```python
from build123d import *

# Parameters (mm, degrees)
SKETCH1_R           = 1.5
SKETCH1_W           = 3
SKETCH1_H           = 3
SKETCH1_W_2         = 94
SKETCH1_H_2         = 20
SKETCH1_H_3         = 10
BOSS_EXTRUDE1_DEPTH = 3


with BuildPart() as part:
    # Sketch1 → Boss-Extrude1 (new body)
    with BuildSketch(Plane(origin=(0, 0, 0), x_dir=(1, 0, 0), z_dir=(0, 1, 0))):
        with BuildLine():
            Line((256, 103), (256, 153))
            Line((256, 153), (253, 153))
            Line((253, 153), (253, 203))
            Line((253, 203), (256, 203))
            Line((256, 203), (256, 237))
            Line((256, 237), (263, 237))
            ThreePointArc((263, 237), (265.121320344, 237.878679656), (266, 240))
            Line((266, 240), (266, 244))
            ThreePointArc((266, 244), (265.121320344, 246.121320344), (263, 247))
            Line((263, 247), (253, 247))
            Line((253, 247), (203, 247))
            Line((203, 247), (203, 250))
            Line((203, 250), (153, 250))
            Line((153, 250), (153, 247))
            Line((153, 247), (103, 247))
            Line((103, 247), (103, 250))
            Line((103, 250), (53, 250))
            Line((53, 250), (53, 247))
            Line((53, 247), (0, 247))
            Line((0, 247), (0, 200))
            Line((0, 200), (3, 200))
            Line((3, 200), (3, 150))
            Line((3, 150), (0, 150))
            Line((0, 150), (0, 100))
            Line((0, 100), (3, 100))
            Line((3, 100), (3, 50))
            Line((3, 50), (0, 50))
            Line((0, 50), (0, 0))
            Line((0, 0), (53, 0))
            Line((53, 0), (53, -3))
            Line((53, -3), (103, -3))
            Line((103, -3), (103, 0))
            Line((103, 0), (153, 0))
            Line((153, 0), (153, -3))
            Line((153, -3), (203, -3))
            Line((203, -3), (203, 0))
            Line((203, 0), (253, 0))
            Line((253, 0), (253, -3))
            Line((253, -3), (256, -3))
            Line((256, -3), (256, 0))
            Line((256, 0), (256, 43))
            Line((256, 43), (262.1, 43))
            Line((262.1, 43), (262.1, 21))
            ThreePointArc((262.1, 21), (262.978679656, 18.878679656), (265.1, 18))
            Line((265.1, 18), (268.1, 18))
            ThreePointArc((268.1, 18), (270.221320344, 18.878679656), (271.1, 21))
            Line((271.1, 21), (271.1, 43))
            Line((271.1, 43), (271.1, 45))
            ThreePointArc((271.1, 45), (269.635533906, 48.535533906), (266.1, 50))
            Line((266.1, 50), (256, 50))
            Line((256, 50), (256, 53))
            Line((256, 53), (253, 53))
            Line((253, 53), (253, 103))
            Line((253, 103), (256, 103))
        make_face()
        with Locations(Location((261, 242, 0), (0, 0, 270))):
            Circle(SKETCH1_R, mode=Mode.SUBTRACT)
        with Locations((266.6, 29.5)):
            Rectangle(SKETCH1_W, SKETCH1_H, mode=Mode.SUBTRACT)
        with Locations((128, 45)):
            Rectangle(SKETCH1_W_2, SKETCH1_H_2, mode=Mode.SUBTRACT)
        with Locations((266.6, 36.5)):
            Rectangle(SKETCH1_W, SKETCH1_H, mode=Mode.SUBTRACT)
        with Locations((251.5, 29.5)):
            Rectangle(SKETCH1_W, SKETCH1_H, mode=Mode.SUBTRACT)
        with Locations((251.5, 36.5)):
            Rectangle(SKETCH1_W, SKETCH1_H, mode=Mode.SUBTRACT)
        Polygon((184, 35), (234, 35), (237, 35), (237, 45), (234, 45), (234, 55), (184, 55), align=None, mode=Mode.SUBTRACT)
        with Locations((76.5, 40)):
            Rectangle(SKETCH1_W, SKETCH1_H_3, mode=Mode.SUBTRACT)
        Polygon((184, 103.5), (234, 103.5), (237, 103.5), (237, 113.5), (234, 113.5), (234, 123.5), (184, 123.5), align=None, mode=Mode.SUBTRACT)
        with Locations((179.5, 40)):
            Rectangle(SKETCH1_W, SKETCH1_H_3, mode=Mode.SUBTRACT)
        with Locations((128, 113.5)):
            Rectangle(SKETCH1_W_2, SKETCH1_H_2, mode=Mode.SUBTRACT)
        with Locations((76.5, 108.5)):
            Rectangle(SKETCH1_W, SKETCH1_H_3, mode=Mode.SUBTRACT)
        with Locations((128, 182)):
            Rectangle(SKETCH1_W_2, SKETCH1_H_2, mode=Mode.SUBTRACT)
        with Locations((179.5, 108.5)):
            Rectangle(SKETCH1_W, SKETCH1_H_3, mode=Mode.SUBTRACT)
        Polygon((184, 172), (234, 172), (237, 172), (237, 182), (234, 182), (234, 192), (184, 192), align=None, mode=Mode.SUBTRACT)
        with Locations((76.5, 177)):
            Rectangle(SKETCH1_W, SKETCH1_H_3, mode=Mode.SUBTRACT)
        with Locations((179.5, 177)):
            Rectangle(SKETCH1_W, SKETCH1_H_3, mode=Mode.SUBTRACT)
        Polygon((22, 35), (72, 35), (72, 55), (22, 55), (22, 45), (19, 45), (19, 35), align=None, mode=Mode.SUBTRACT)
        Polygon((22, 103.5), (72, 103.5), (72, 123.5), (22, 123.5), (22, 113.5), (19, 113.5), (19, 103.5), align=None, mode=Mode.SUBTRACT)
        Polygon((22, 172), (72, 172), (72, 192), (22, 192), (22, 182), (19, 182), (19, 172), align=None, mode=Mode.SUBTRACT)
    extrude(amount=BOSS_EXTRUDE1_DEPTH)


solid = part.part
```
Input: part model. Units: mm. Frame: model coordinates. Coordinates: 2 decimals unless noted, no trailing zeros. Loops run counter-clockwise (first coordinate to the right, second up) from the corner with the lowest first, then second, coordinate; pieces in that order, holes last. Notation, with made-up numbers: (25, 77) - (52, 77) arc R24 ccw to (52, 102) - close; hole circle Ø4 at (50.25, 74). An arc over 180 degrees is marked (long way). Answer in a Markdown table with one row per item.
(1) Material intervals for L1, parallel to Z at x = 261, y = 2; L2, parallel to Z at x = 224, y = 2.8; L3, parallel to Z at x = 155, y = 0.85, sorted ascending. Write a range as from..to.
Model answer:
| item | result |
|---|---|
| L1 | z = -247..-243.5, -240.5..-237, -50..-43 |
| L2 | z = -247..-192, -172..-123.5, -103.5..-55, -35..0 |
| L3 | z = -250..-192, -172..-123.5, -103.5..-55, -35..3 |
(2) Pin query (flat end, axial travel): P1, Ø0.9, axis at y = 1, z = -110.5, coming from the +X side; P2, Ø0.9, axis at x = 261, y = 1.5, coming from the -Z side; P3, Ø8, axis at x = 54, z = -195.5, coming from the -Y side; P4, Ø1.5, axis at y = 1.5, z = -178.5, coming from the -X side. Return the tip coordinate at first contact, or that it passes through.
Model answer:
| item | result |
|---|---|
| P1 | stops at x = 256 |
| P2 | stops at z = -247 |
| P3 | stops at y = 0 |
| P4 | stops at x = 3 |
(3) Cut plane A-A on x = 26. Output: boundary loops of the cut face in (y, z), plus the area to 3 significant figures.
Model answer:
| item | result |
|---|---|
| outline | (0, -247) - (3, -247) - (3, -192) - (0, -192) - close; (0, -172) - (3, -172) - (3, -123.5) - (0, -123.5) - close; (0, -103.5) - (3, -103.5) - (3, -55) - (0, -55) - close; (0, -35) - (3, -35) - (3, 0) - (0, 0) - close |
| area | 561 mm² |
(4) Cut plane C-C on x = 91.5. Output: boundary loops of the cut face in (y, z).
Model answer:
| item | result |
|---|---|
| outline | (0, -250) - (3, -250) - (3, -192) - (0, -192) - close; (0, -172) - (3, -172) - (3, -123.5) - (0, -123.5) - close; (0, -103.5) - (3, -103.5) - (3, -55) - (0, -55) - close; (0, -35) - (3, -35) - (3, 3) - (0, 3) - close |
(5) Cut plane D-D on x = 241.5. Output: boundary loops of the cut face in (y, z).
Model answer:
| item | result |
|---|---|
| outline | (0, -247) - (3, -247) - (3, 0) - (0, 0) - close |
(6) Cut plane B-B on y = 2. Count the separate pieces of the cut face and the enclosed holes in it, plus the area to 3 significant figures.
Model answer:
| item | result |
|---|---|
| separate pieces | 1 |
| enclosed holes | 20 |
| area | 51,600 mm² |
